```python
from build123d import *

# Parameters (mm, degrees)
BOSS_EXTRU_1_DEPTH           = 3
ESQUISSE2_R                  = 14.1
ENL_V_MAT_EXTRU_1_DEPTH      = 3
CONG_1_R                     = 20
ENL_V_MAT_EXTRU_2_DEPTH      = 3
R_P_TITION_CIRCULAIRE1_COUNT = 8


with BuildPart() as part:
    # Esquisse1 → Boss.-Extru.1 (new body)
    with BuildSketch(Plane.XY):
        Polygon((0, 0), (0, 35), (-3, 35), (-3, 65), (0, 65), (0, 100), (35, 100), (35, 103), (65, 103), (65, 100), (100, 100), (100, 65), (103, 65), (103, 35), (100, 35), (100, 0), (65, 0), (65, -3), (35, -3), (35, 0), align=None)
    extrude(amount=BOSS_EXTRU_1_DEPTH)

    # Esquisse2 → Enlèv. mat.-Extru.1 (cut)
    with BuildSketch(Plane.XY.offset(3)):
        with Locations((50, 50)):
            Circle(ESQUISSE2_R)
    extrude(amount=-ENL_V_MAT_EXTRU_1_DEPTH, mode=Mode.SUBTRACT)

    # Congé1
    cong_1_edges = [part.edges().sort_by_distance(p)[0] for p in [
        (0, 0, 1.5),
        (0, 100, 1.5),
        (100, 100, 1.5),
        (100, 0, 1.5),
    ]]
    fillet(cong_1_edges, radius=CONG_1_R)

    # Esquisse4 → Enlèv. mat.-Extru.2 (cut)
    with BuildSketch(Plane.XY.offset(3)):
        with BuildLine():
            Line((52.544857736, 93.542670146), (52.544857736, 77.800875632))
            ThreePointArc((52.544857736, 77.800875632), (50.044857736, 75.300875632), (47.544857736, 77.800875632))
            Line((47.544857736, 77.800875632), (47.544857736, 93.542670146))
            ThreePointArc((47.544857736, 93.542670146), (50.044857736, 96.042670146), (52.544857736, 93.542670146))
        make_face()
    enl_v_mat_extru_2 = extrude(amount=-ENL_V_MAT_EXTRU_2_DEPTH, mode=Mode.SUBTRACT)

    # Répétition circulaire1: Enlèv. mat.-Extru.2 ×8 about axis
    r_p_tition_circulaire1_axis = Axis((50, 50, 0), (0, 0, 1))
    for i in range(1, R_P_TITION_CIRCULAIRE1_COUNT):
        add(enl_v_mat_extru_2.rotate(r_p_tition_circulaire1_axis, i * 360 / R_P_TITION_CIRCULAIRE1_COUNT), mode=Mode.SUBTRACT)


solid = part.part
```
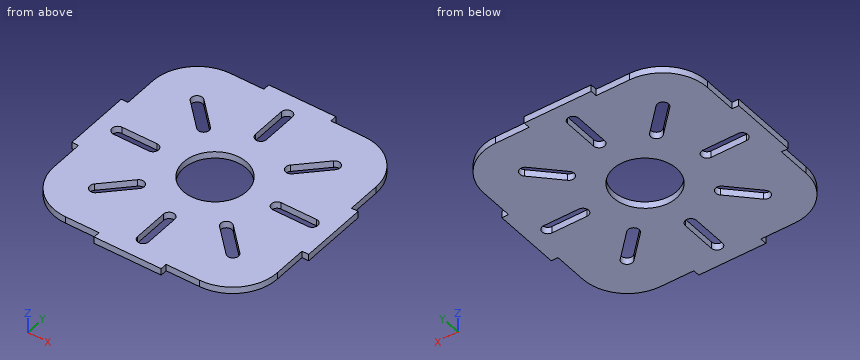
Verification items for the finished model (mm, model axes). Round coordinates to 2 decimals unless told otherwise and drop trailing zeros. Write each loop counter-clockwise with the first axis right and the second up, starting at its lowest first coordinate (ties: lowest second). Pieces come first, ordered by that corner, then holes. Notation, with made-up numbers: (-28.75, 33.25) - (-4.75, 33.25) arc R26 ccw to (-4.75, 67.25) - close; hole circle Ø9 at (12, 18). An arc over 180 degrees is marked (long way). Answer as a JSON object with one key per item and string values. Group by question number.
Q1. Go/stop test with flat-tipped pins: pin 1 Ø1.5 at (x, y) = (69, 79) entering from -Z; pin 2 Ø1.5 at (x, z) = (102, 2) entering from -Y; pin 3 Ø0.9 at (y, z) = (102, 1) entering from -X; pin 4 Ø0.9 at (x, z) = (-2, 1.5) entering from +Y. Record where each tip stops, or that it passes through.
Q2. Section check B-B, the plane y = 50. Enter the section's corners in (x, z), plus the area to 3 significant figures.
Q3. Section check A-A, the plane x = 41. Enter the section's corners in (y, z), plus the area to 3 significant figures.
Q4. Section check C-C, the plane z = 0.5. Give the number of separate pieces and of enclosed holes in the cut face, plus the area to 3 significant figures.
Q5. Section check D-D, the plane x = 14.5. Enter the section's corners in (y, z).
Q6. Thickness scan on line 1 (Y direction, x = 50, z = 1.5); line 2 (Y direction, x = 51, z = 0.55); line 3 (X direction, y = 30, z = 1.5). Record the ranges inside material, lowest first.
Found:
{
 "1": {"pin 1": "stops at z = 0", "pin 2": "stops at y = 35", "pin 3": "stops at x = 35", "pin 4": "stops at y = 65"},
 "2": {"outline": "(-3, 0) - (3.96, 0) - (3.96, 3) - (-3, 3) - close; (24.7, 0) - (35.9, 0) - (35.9, 3) - (24.7, 3) - close; (64.1, 0) - (75.3, 0) - (75.3, 3) - (64.1, 3) - close; (96.04, 0) - (103, 0) - (103, 3) - (96.04, 3) - close", "area": "109 mm^2"},
 "3": {"outline": "(-3, 0) - (39.15, 0) - (39.15, 3) - (-3, 3) - close; (60.85, 0) - (103, 0) - (103, 3) - (60.85, 3) - close", "area": "253 mm^2"},
 "4": {"separate pieces": "1", "enclosed holes": "9", "area": "8,610 mm^2"},
 "5": {"outline": "(0.77, 0) - (47.54, 0) - (47.54, 3) - (0.77, 3) - close; (52.54, 0) - (99.23, 0) - (99.23, 3) - (52.54, 3) - close"},
 "6": {"line 1": "y = -3 to 3.96, 24.7 to 35.9, 64.1 to 75.3, 96.04 to 103", "line 2": "y = -3 to 4.19, 24.47 to 35.94, 64.06 to 75.49, 95.85 to 103", "line 3": "x = 0 to 26.4, 32.78 to 67.15, 73.47 to 100"}
}
